```python
from build123d import *

# Parameters (mm, degrees)
SKETCH1_W           = 33.5
SKETCH1_H           = 19.083452378
SKETCH1_R           = 1.5
SKETCH1_W_2         = 4.666904756
SKETCH1_H_2         = 4.666904756
BOSS_EXTRUDE1_DEPTH = 2
SKETCH1_3_W         = 4.666904756
SKETCH1_3_H         = 4.666904756
BOSS_EXTRUDE2_DEPTH = 49
SKETCH3_R           = 2.15
CUT_EXTRUDE1_DEPTH  = 2.25


with BuildPart() as part:
    # Sketch1 → Boss-Extrude1 (new body)
    # profile 1 of 5: a face of its own
    with BuildSketch(Plane(origin=(0, 0, 0), x_dir=(0, 0, -1), z_dir=(1, 0, 0))):
        with Locations((0, 7.208273811)):
            Rectangle(SKETCH1_W, SKETCH1_H)
        with Locations((8.485281374, 8.485281374)):
            Circle(SKETCH1_R, mode=Mode.SUBTRACT)
        with Locations((-8.485281374, 8.485281374)):
            Circle(SKETCH1_R, mode=Mode.SUBTRACT)
        with Locations((-14.75, 0)):
            Circle(SKETCH1_R, mode=Mode.SUBTRACT)
        with Locations((14.75, 0)):
            Circle(SKETCH1_R, mode=Mode.SUBTRACT)
        with Locations((0, 14.75)):
            Circle(SKETCH1_R, mode=Mode.SUBTRACT)
    # profile 2 of 5: a face of its own
    with BuildSketch(Plane(origin=(0, 0, 0), x_dir=(0, 0, -1), z_dir=(1, 0, 0))):
        Rectangle(SKETCH1_W_2, SKETCH1_H_2)
    # profile 3 of 5: a face of its own
    with BuildSketch(Plane(origin=(0, 0, 0), x_dir=(0, 0, -1), z_dir=(1, 0, 0))):
        with BuildLine():
            ThreePointArc((-2.333452378, 2.333452378), (-3.3, 0), (-2.333452378, -2.333452378))
            Line((-2.333452378, -2.333452378), (-2.333452378, 2.333452378))
        make_face()
    # profile 4 of 5: a face of its own
    with BuildSketch(Plane(origin=(0, 0, 0), x_dir=(0, 0, -1), z_dir=(1, 0, 0))):
        with BuildLine():
            ThreePointArc((2.333452378, 2.333452378), (0, 3.3), (-2.333452378, 2.333452378))
            Line((-2.333452378, 2.333452378), (2.333452378, 2.333452378))
        make_face()
    # profile 5 of 5: a face of its own
    with BuildSketch(Plane(origin=(0, 0, 0), x_dir=(0, 0, -1), z_dir=(1, 0, 0))):
        with BuildLine():
            Line((2.333452378, 2.333452378), (2.333452378, -2.333452378))
            ThreePointArc((2.333452378, -2.333452378), (3.048802457, -1.262855327), (3.3, 0))
            ThreePointArc((3.3, 0), (3.048802457, 1.262855327), (2.333452378, 2.333452378))
        make_face()
    extrude(amount=BOSS_EXTRUDE1_DEPTH)

    # Sketch1_3 → Boss-Extrude2 (add)
    with BuildSketch(Plane(origin=(0, 0, 0), x_dir=(0, 0, -1), z_dir=(1, 0, 0))):
        Rectangle(SKETCH1_3_W, SKETCH1_3_H)
        with BuildLine():
            ThreePointArc((-2.333452378, 2.333452378), (-3.3, 0), (-2.333452378, -2.333452378))
            Line((-2.333452378, -2.333452378), (-2.333452378, 2.333452378))
        make_face()
        with BuildLine():
            ThreePointArc((2.333452378, 2.333452378), (0, 3.3), (-2.333452378, 2.333452378))
            Line((-2.333452378, 2.333452378), (2.333452378, 2.333452378))
        make_face()
        with BuildLine():
            Line((2.333452378, 2.333452378), (2.333452378, -2.333452378))
            ThreePointArc((2.333452378, -2.333452378), (3.048802457, -1.262855327), (3.3, 0))
            ThreePointArc((3.3, 0), (3.048802457, 1.262855327), (2.333452378, 2.333452378))
        make_face()
    extrude(amount=BOSS_EXTRUDE2_DEPTH)

    # Sketch3 → Cut-Extrude1 (cut)
    with BuildSketch(Plane(origin=(49, 0, 0), x_dir=(0, 0, -1), z_dir=(1, 0, 0))):
        Circle(SKETCH3_R)
    extrude(amount=-CUT_EXTRUDE1_DEPTH, mode=Mode.SUBTRACT)


solid = part.part
```
The model under review builds one solid part; all positions refer to its coordinate system, in mm. A direction names the side the tool comes from. Coordinates: 2 decimals unless noted, no trailing zeros. Order: outer loops, then holes, each group sorted by start corner. A loop starts at its lowest first (then second) coordinate and runs counter-clockwise, first axis right, second up. Notation, with made-up numbers: M 49,-30.5 L 78,-30.5 A8 ccw 78,-16.5 Z; hole C 53,79 d1. An arc over 180 degrees is marked long. One line per question, with ' | ' between items.
(1) For probe 1 along Y at (x, z) = (0.55, -14.75); probe 2 along X at (y, z) = (10.5, -2); probe 3 along Z at (x, y) = (43.5, -0.25), list the stretches that pass through material, from the lowest coordinate up. Write a range as from..to.
Geometry results:
probe 1: y = -2.33..-1.5, 1.5..16.75 | probe 2: x = 0..2 | probe 3: z = -3.29..3.29
(2) Insertion check: pin 1 (3.5 mm diameter, centred on y = 0, z = 0, fed in from +X); pin 2 (2 mm diameter, centred on y = -1, z = 1, fed in from +X); pin 3 (5 mm diameter, centred on y = 8.49, z = 8.49, fed in from +X). Each pin has a flat end and moves straight along its axis. Give the tip position at first contact, or say it passes through.
Geometry results:
pin 1: stops at x = 46.75 | pin 2: stops at x = 49 | pin 3: stops at x = 2
(3) Machinability: for faces 5 (the face through (0.99, 0.07, -13.25)), 6 (the face through (47.89, 0.09, 2.15)), which of the approach directions +Z, -Z, +X, -X, +Y, -Y give a long, thin tool a straight path to every point of the face, cutting with its end or side? Answer none if there is none.
Geometry results:
face 5: +X, -X | face 6: +X
(4) Add section B-B, the plane z = 14.75. Write out the cut boundary in (x, y), then the cut area to 3 significant figures.
Geometry results:
outline: M 0,-2.33 L 2,-2.33 L 2,-1.5 L 0,-1.5 Z; M 0,1.5 L 2,1.5 L 2,16.75 L 0,16.75 Z | area: 32.2 mm²
(5) Add section C-C, the plane x = 11.5. Write out the cut boundary in (y, z), then the cut area to 3 significant figures.
Geometry results:
outline: M -2.33,-2.33 A3.3 ccw long -2.33,2.33 Z | area: 31.1 mm²
(6) Add section D-D, the plane z = 0. Write out the cut boundary in (x, y).
Geometry results:
outline: M 0,-2.33 L 49,-2.33 L 49,-2.15 L 46.75,-2.15 L 46.75,2.15 L 49,2.15 L 49,3.3 L 2,3.3 L 2,13.25 L 0,13.25 Z; M 0,16.25 L 2,16.25 L 2,16.75 L 0,16.75 Z
(7) The part is to be moulded in two halves that separate along Z. For faces 1 (the face through (0.986, 13.286, 0.325)), 2 (the face through (1, 7, 16.75)), 3 (the face through (0.99, 9.75, -9.29)), 4 (the face through (49, 2.4, 0)), say which applies: +Z half, -Z half, draft (parallel to the pull), parting line (faces both ways), or undercut.
Geometry results:
face 1: undercut | face 2: +Z half | face 3: undercut | face 4: draft
(8) Add section A-A, the plane y = 14.75. Write out the cut boundary in (x, z), then the cut area to 3 significant figures.
Geometry results:
outline: M 0,-16.75 L 2,-16.75 L 2,-1.5 L 0,-1.5 Z; M 0,1.5 L 2,1.5 L 2,16.75 L 0,16.75 Z | area: 61.0 mm²
